Check sheet for the modelled part. Datum: model origin and axes. Units: mm. Give positions to 0.01 mm unless a question says otherwise; leave off trailing zeros. Order: outer loops, then holes, each group sorted by start corner. A loop starts at its lowest first (then second) coordinate and runs counter-clockwise, first axis right, second up. Notation, with made-up numbers: (-21.5, 57.25) -> (1.5, 57.25) arc R11 cw to (1.5, 61.25) -> close; hole circle Ø11 at (-11.5, 11.25). An arc over 180 degrees is marked (long way). Answer in a Markdown table with one row per item. Add a question column.
(1) Cross-section at B-B (x = -117.5). Record the cut outline in (y, z), then the cut area to 3 significant figures.
(2) Cross-section at C-C (z = -75). Record the cut outline in (x, y).
(3) Thickness scan on L1, parallel to X at y = 0.85, z = -25; L2, parallel to X at y = 0.7, z = 0; L3, parallel to X at y = 1.25, z = -3. Record the ranges inside material, lowest first. Write a range as [from, to].
(4) Cross-section at A-A (y = 1.9). State how many separate pieces and enclosed holes the cut face has, then the cut area to 3 significant figures.
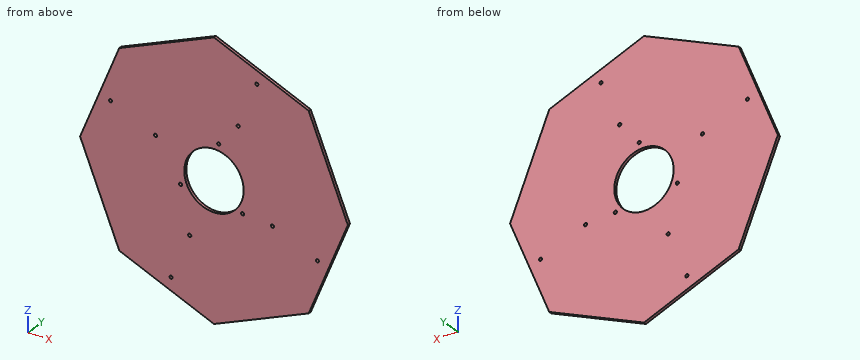
Autodesk Inventor part; units mm, degrees
ref_plane "YZ Plane" through (0, 0, 0) normal (1, 0, 0) x (0, 1, 0)
ref_plane "XZ Plane" through (0, 0, 0) normal (0, 1, 0) x (-1, 0, 0)
ref_plane "XY Plane" through (0, 0, 0) normal (0, 0, 1) x (1, 0, 0)
sketch "スケッチ1" plane through (0, 0, 0) normal (0, 1, 0) x (-1, 0, 0)
  circle A0 centre (0, 0) radius 135.299
  line L0 (0, 0) -> (135.299, 0)
  line L1 (0, 0) -> (95.6709, -95.6709)
  line L2 (0, 0) -> (0, -135.299)
  line L3 (0, 0) -> (-95.6709, -95.6709)
  line L4 (0, 0) -> (-135.299, 0)
  line L5 (0, 0) -> (-95.6709, 95.6709)
  line L6 (0, 0) -> (0, 135.299)
  line L7 (0, 0) -> (95.6709, 95.6709)
  line L8 (135.299, 0) -> (95.6709, -95.6709)
  line L9 (95.6709, 95.6709) -> (135.299, 0)
  line L10 (0, 135.299) -> (95.6709, 95.6709)
  line L11 (-95.6709, 95.6709) -> (0, 135.299)
  line L12 (-135.299, 0) -> (-95.6709, 95.6709)
  line L13 (-95.6709, -95.6709) -> (-135.299, 0)
  line L14 (0, -135.299) -> (-95.6709, -95.6709)
  line L15 (95.6709, -95.6709) -> (0, -135.299)
  circle A1 centre (0, 0) radius 125
  point P0 (0, 135.299)
  point P1 (-95.6709, 95.6709)
  point P2 (-135.299, 0)
  point P3 (95.6709, -95.6709)
  dimension "d3" = 360
  dimension "d7" = 360
  dimension "d57" = 250
extrude "押し出し1" add sketch "スケッチ1" along normal blind 3 contours L8 A1 L0 | L0 A1 L9 | L9 A1 L7 | L7 A1 L10 | L15 A1 L1 | L1 A1 L8 | A1 L1 L0 | L0 L7 A1 | L10 A1 L6 | L6 A1 L11 | L7 L6 A1 | L14 A1 L2 | L2 A1 L15 | A1 L2 L1 | L2 A1 L3 | L3 A1 L4 | L4 A1 L5 | L5 A1 L6 | L11 A1 L5 | L5 A1 L12 | L13 A1 L3 | L3 A1 L14 | A1 L13 L4 | L4 L12 A1
sketch "スケッチ2" plane through (0, 3, 0) normal (0, 1, 0) x (1, 0, 0)
  circle A0 centre (0, 0) radius 64
  circle A1 centre (0, 0) radius 36.5
  line L0 (0, 0) -> (-59.1283, 24.4917)
  line L1 (-95.6709, 95.6709) -> (-135.299, 0)
  line L2 (0, 0) -> (-135.299, 0)
  point P0 (-33.7216, 13.9679)
  point P1 (4.7642, -36.1877)
  point P2 (28.9574, 22.2198)
  dimension "d11" = 128
  dimension "d12" = 73
  dimension "d13" = 22.5
  dimension "d16" = 360
hole "穴1" at (-33.7216, 3, -13.9679) at (4.7642, 3, 36.1877) at (28.9574, 3, -22.2198) direction (0, -1, 0) diameter 3.2 end through all
sketch "スケッチ3" plane through (0, 3, 0) normal (0, 1, 0) x (1, 0, 0)
  circle A0 centre (0, 0) radius 64
  line L0 (0, 0) -> (-59.1283, -24.4917)
  line L1 (0, 0) -> (-29.4133, 0)
  point P0 (-59.1283, -24.4917)
  point P1 (24.4917, -59.1283)
  point P2 (59.1283, 24.4917)
  point P3 (-24.4917, 59.1283)
  dimension "d25" = 128
  dimension "d28" = 360
  dimension "d56" = 22.5
hole "穴2" at (-59.1283, 3, 24.4917) at (24.4917, 3, 59.1283) at (59.1283, 3, -24.4917) at (-24.4917, 3, -59.1283) direction (0, -1, 0) diameter 3.2 end through all
sketch "スケッチ4" plane through (0, 0, 0) normal (0, -1, 0) x (1, 0, 0)
  circle A0 centre (-33.7216, -13.9679) radius 1.6
  circle A1 centre (-33.7216, -13.9679) radius 3
  circle A2 centre (28.9574, -22.2198) radius 3
  circle A3 centre (4.7642, 36.1877) radius 3
  circle A4 centre (-24.4917, -59.1283) radius 1.6
  circle A5 centre (-24.4917, -59.1283) radius 3.9
  circle A6 centre (59.1283, -24.4917) radius 3.9
  circle A7 centre (24.4917, 59.1283) radius 3.9
  circle A8 centre (-59.1283, 24.4917) radius 3.9
  point P0 (0, 0)
  point P1 (0, 0)
  point P2 (0, 0)
  dimension "d37" = 6
  dimension "d40" = 360
  dimension "d42" = 7.8
  dimension "d45" = 360
extrude "押し出し2" [suppressed]
sketch "スケッチ5" plane through (0, 0, 0) normal (0, -1, 0) x (1, 0, 0)
  circle A0 centre (59.1283, -24.4917) radius 1.6
  circle A1 centre (59.1283, -24.4917) radius 3.9
  circle A2 centre (24.4917, 59.1283) radius 3.9
  circle A3 centre (-59.1283, 24.4917) radius 3.9
  circle A4 centre (-24.4917, -59.1283) radius 3.9
  point P0 (0, 0)
  dimension "d49" = 7.8
  dimension "d52" = 360
extrude "押し出し3" [suppressed]
sketch "スケッチ6" plane through (0, 0, 0) normal (0, -1, 0) x (1, 0, 0)
  line L0 (0, 0) -> (115.4849, 47.8354)
  line L1 (95.6709, 95.6709) -> (135.299, 0)
  line L2 (0, 135.299) -> (95.6709, 95.6709)
  line L3 (58.7953, 110.9452) -> (-120.0247, 36.8755)
  line L4 (-135.299, 0) -> (-95.6709, 95.6709)
  line L5 (-95.6709, 95.6709) -> (0, 135.299)
  line L6 (135.299, 0) -> (95.6709, -95.6709)
  line L7 (120.0247, -36.8755) -> (-58.7953, -110.9452)
  line L8 (0, -135.299) -> (-95.6709, -95.6709)
  line L9 (95.6709, -95.6709) -> (0, -135.299)
  line L10 (0, 0) -> (-30.6147, 73.9104)
  point P0 (43.2957, 104.525)
  point P1 (-104.525, 43.2957)
  point P2 (104.525, -43.2957)
  point P3 (-43.2957, -104.525)
  dimension "d58" = 80
  dimension "d59" = 80
  dimension "d60" = 80
hole "穴3" at (43.2957, 0, 104.525) at (-104.525, 0, 43.2957) at (104.525, 0, -43.2957) at (-43.2957, 0, -104.525) direction (0, 1, 0) diameter 3.1 end through all
sketch "スケッチ7" plane through (0, 3, 0) normal (0, 1, 0) x (1, 0, 0)
  circle A0 centre (0, 0) radius 30
  dimension "d68" = 60
extrude "押し出し4" cut sketch "スケッチ7" against normal blind 10
properties part number "Largebaseplate" material "アルミニウム 6061"
Answer below:
| question | item | result |
|---|---|---|
| 1 | outline | (0, -42.97) -> (3, -42.97) -> (3, 42.97) -> (0, 42.97) -> close |
| 1 | area | 258 mm² |
| 2 | outline | (-104.23, 0) -> (104.23, 0) -> (104.23, 3) -> (-104.23, 3) -> close |
| 3 | L1 | x = [-124.94, -16.58], [16.58, 57.61], [60.65, 124.94] |
| 3 | L2 | x = [-135.3, -30], [30, 135.3] |
| 3 | L3 | x = [-134.06, -29.85], [29.85, 134.06] |
| 4 | separate pieces | 1 |
| 4 | enclosed holes | 12 |
| 4 | area | 48,900 mm² |
